Here's the drawing with two shaded views (mm, measured from the low corner). I have some questions. Coordinates: 2 decimals unless noted, no trailing zeros. Order: outer loops, then holes, each group sorted by start corner. A loop starts at its lowest first (then second) coordinate and runs counter-clockwise, first axis right, second up. Notation, with made-up numbers: (85.25, 26) -> (98.25, 26) arc R32 cw to (98.25, 52) -> close; hole circle Ø8 at (35, 26). An arc over 180 degrees is marked (long way). Answer as a JSON object with one key per item and string values. Group by question number.
(1) I want a section at D-D, the plane z = 62.5. List the corners of the cut face in (x, y) for me, plus the area to 3 significant figures.
(2) I want a section at A-A, the plane z = 112.5. List the corners of the cut face in (x, y) for me, plus the area to 3 significant figures.
(3) I need wall thicknesses on line 1 (Y direction, x = 0.7, z = 63.5) (1 decimal); line 2 (Y direction, x = 4.3, z = 65.5) (1 decimal); line 3 (Z direction, x = 4.85, y = 109.5) (1 decimal). Which ranges of each line are inside material? Lowest first, please.
(4) I want a section at B-B, the plane x = 0.95. List the corners of the cut face in (y, z) for me.
(5) For pin 1 (6.5 mm diameter, centred on y = 37.5, z = 105.8, fed in from +X); pin 2 (3 mm diameter, centred on x = 4, z = 38, fed in from +Y); pin 3 (2 mm diameter, centred on x = 4, y = 111.5, fed in from -Z); pin 4 (1.5 mm diameter, centred on x = 4, z = 82, fed in from +Y), each with a flat end and sliding along its axis, tell me the tip position at first contact or that it passes through.
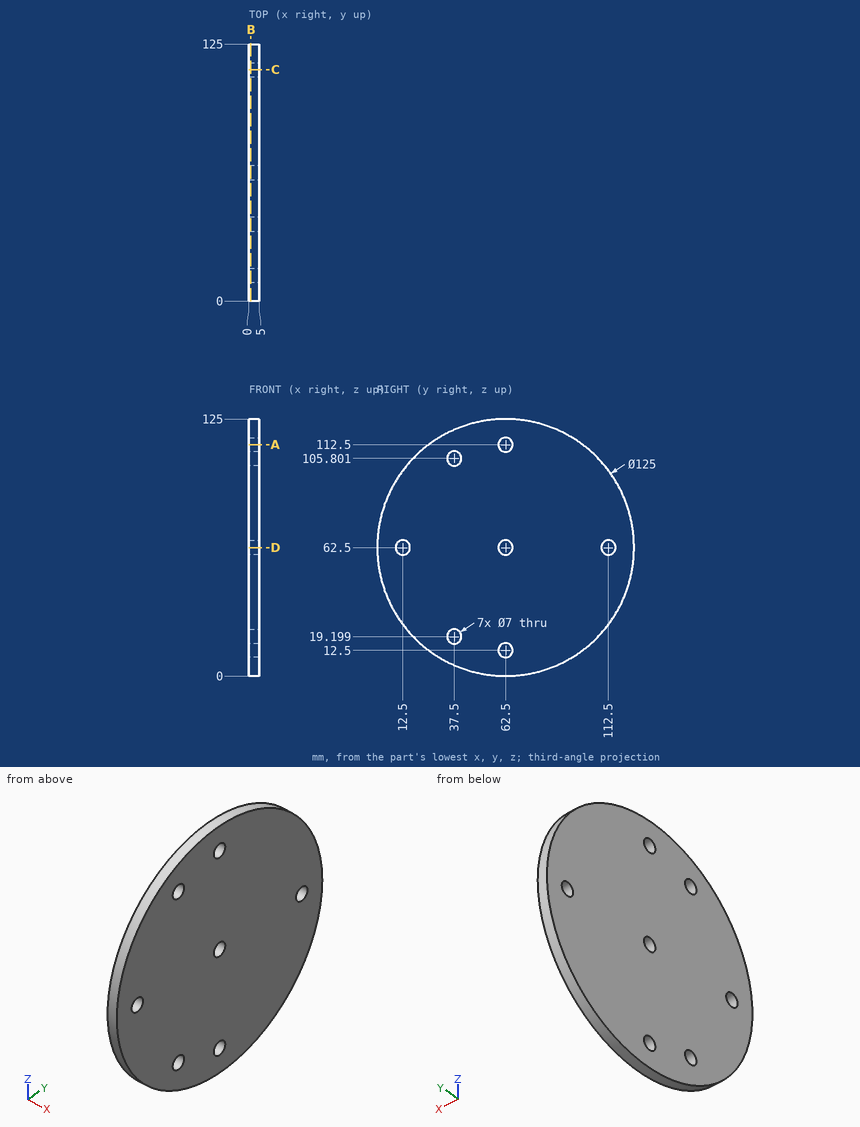
Computed values:
{
 "1": {"outline": "(0, 0) -> (5, 0) -> (5, 9) -> (0, 9) -> close; (0, 16) -> (5, 16) -> (5, 59) -> (0, 59) -> close; (0, 66) -> (5, 66) -> (5, 109) -> (0, 109) -> close; (0, 116) -> (5, 116) -> (5, 125) -> (0, 125) -> close", "area": "520 mm2"},
 "2": {"outline": "(0, 25) -> (5, 25) -> (5, 59) -> (0, 59) -> close; (0, 66) -> (5, 66) -> (5, 100) -> (0, 100) -> close", "area": "340 mm2"},
 "3": {"line 1": "y = 0 to 9.1, 15.9 to 59.1, 65.9 to 109.1, 115.9 to 125", "line 2": "y = 0.1 to 10.7, 14.3 to 60.7, 64.3 to 110.7, 114.3 to 124.9", "line 3": "z = 21.3 to 60.7, 64.3 to 103.7"},
 "4": {"outline": "circle Ø125 at (62.5, 62.5); hole circle Ø7 at (12.5, 62.5); hole circle Ø7 at (37.5, 19.2); hole circle Ø7 at (37.5, 105.8); hole circle Ø7 at (62.5, 12.5); hole circle Ø7 at (62.5, 62.5); hole circle Ø7 at (62.5, 112.5); hole circle Ø7 at (112.5, 62.5)"},
 "5": {"pin 1": "passes through", "pin 2": "stops at y = 120.61", "pin 3": "stops at z = 22.47", "pin 4": "stops at y = 122.12"}
}
